Answer from the drawing. Dimensions are ordinates in mm from the lowest x, y and z of the part. A direction names the side the tool comes from. Give positions to 0.01 mm unless a question says otherwise; leave off trailing zeros. Loops run counter-clockwise (first coordinate to the right, second up) from the corner with the lowest first, then second, coordinate; pieces in that order, holes last.
(1) Find section B-B, the plane x = 0.85. Write down the section's boundary in (y, z).
(2) Find section C-C, the plane y = 4.6. Write down the section's boundary in (x, z).
(3) Which of the six approach directions +Z, -Z, +X, -X, +Y, -Y give full straight-line access (tool end or side, diameter ignored) to the marked faces 1 and 2?
(4) Straight lines are drawn through the part: probe 1 along X at (y, z) = (4.15, 1.5); probe 2 along Z at (x, y) = (3, 2.6); probe 3 along X at (y, z) = (1.75, 3.25). For each, find the intervals that lie inside material, in ascending order.
(5) Find section D-D, the plane x = 3. Write down the section's boundary in (y, z).
(6) Determine the mould class of the marked faces 3, 4, 5 and 6 for opening direction X: pulls with the +X half, pulls with the -X half, needs draft (parallel to the pull), parting line crosses it, or undercut.
(7) Find section A-A, the plane z = 1.25. Write down the section's boundary in (x, y).
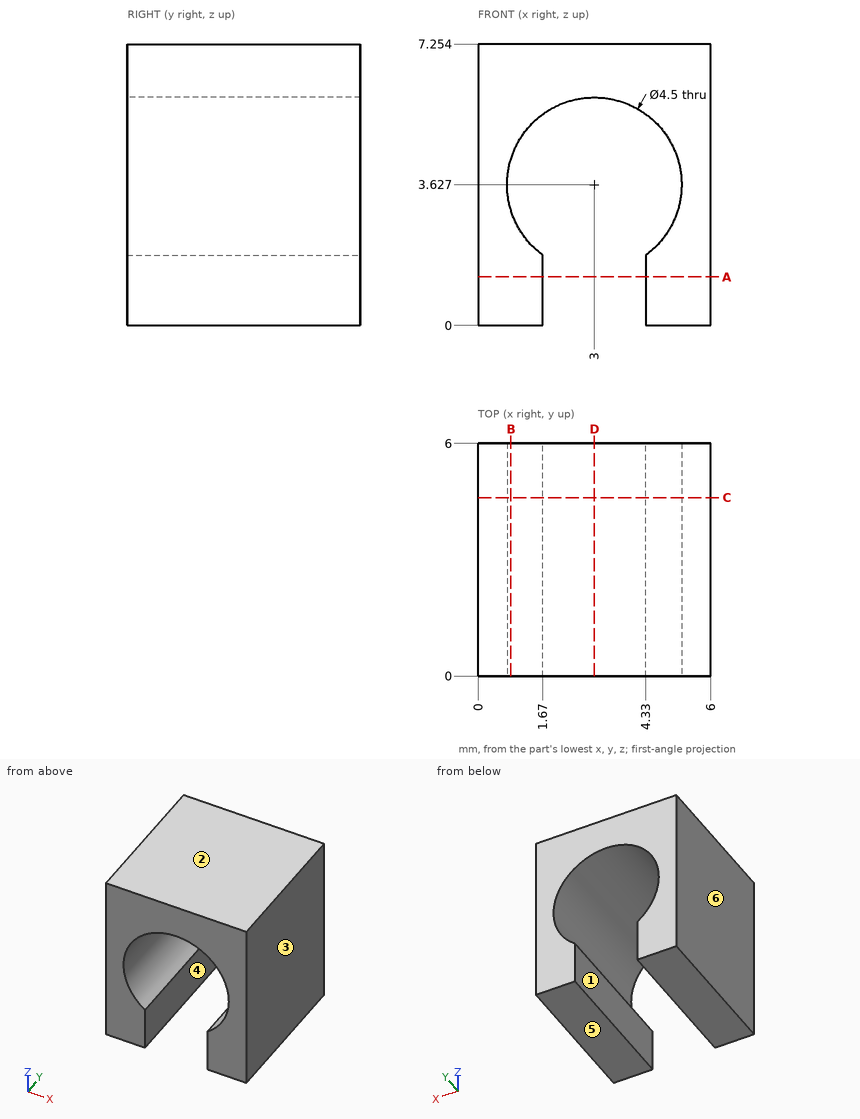
Entries:
1. outline: (0, 0) - (6, 0) - (6, 2.96) - (0, 2.96) - close; (0, 4.29) - (6, 4.29) - (6, 7.25) - (0, 7.25) - close
2. outline: (0, 0) - (1.67, 0) - (1.67, 1.81) arc R2.25 cw (long way) to (4.33, 1.81) - (4.33, 0) - (6, 0) - (6, 7.25) - (0, 7.25) - close
3. face 1: -Z, +Y, -Y
3. face 2: +Z, +X, -X, +Y, -Y
4. probe 1: x = 0 to 1.67, 4.33 to 6
4. probe 2: z = 5.88 to 7.25
4. probe 3: x = 0 to 0.78, 5.22 to 6
5. outline: (0, 5.88) - (6, 5.88) - (6, 7.25) - (0, 7.25) - close
6. face 3: pulls with the +X half
6. face 4: undercut
6. face 5: needs draft
6. face 6: pulls with the -X half
7. outline: (0, 0) - (1.67, 0) - (1.67, 6) - (0, 6) - close; (4.33, 0) - (6, 0) - (6, 6) - (4.33, 6) - close
